Source: three-view drawing plus pictorial views. Frame: mm from the lowest corner of the part. Coordinates: 2 decimals unless noted, no trailing zeros. Loops run counter-clockwise (first coordinate to the right, second up) from the corner with the lowest first, then second, coordinate; pieces in that order, holes last. Notation, with made-up numbers: M -38,-27.5 L -23,-27.5 A20 cw -23,-22.5 Z; hole C 39.5,-6 d11. An arc over 180 degrees is marked long. Use a Markdown table: item, result. Add a question column.
1. Pin query (flat end, axial travel): pin 1 (0.5 mm diameter, centred on x = 79.5, z = 0.5, fed in from -Y). Return the tip coordinate at first contact, or that it passes through.
2. Section B-B on y = 25. Output: boundary loops of the cut face in (x, z).
3. Section C-C on x = 54. Output: boundary loops of the cut face in (y, z), then the cut area to 3 significant figures.
4. Section A-A on z = 0.45. Output: boundary loops of the cut face in (x, y).
5. Line query: L1, parallel to Y at x = 3, z = 0.6; L2, parallel to Y at x = 81, z = 0.15; L3, parallel to Y at x = 14, z = 0.7. Output: solid intervals per line, ascending. Write a range as [from, to].
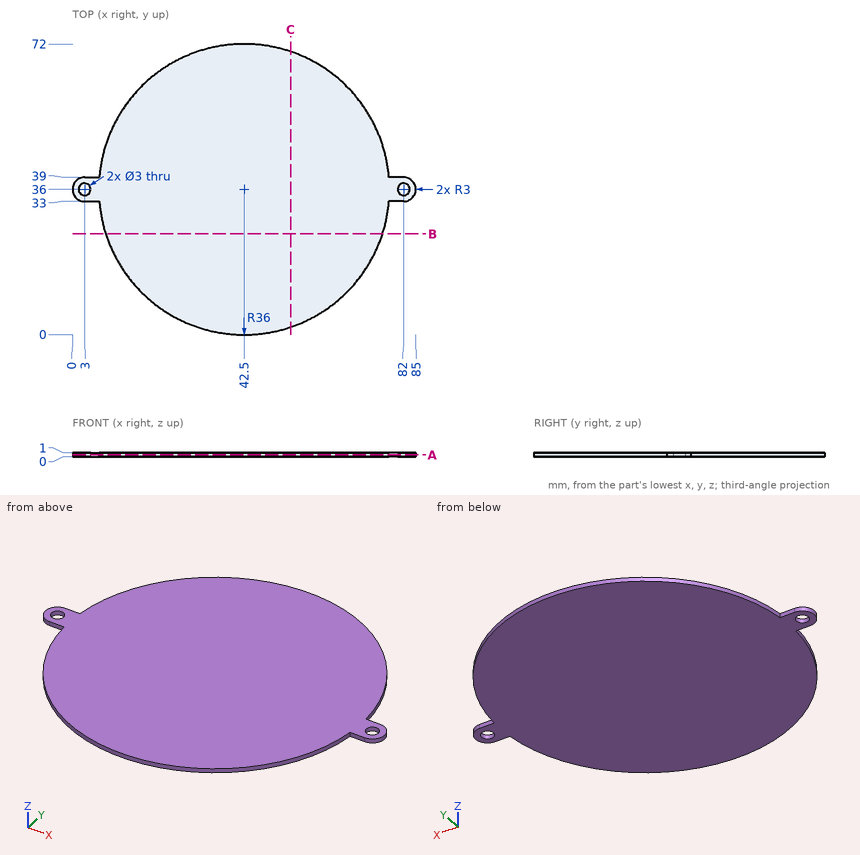
Answers below:
| question | item | result |
|---|---|---|
| 1 | pin 1 | stops at y = 33 |
| 2 | outline | M 8.22,0 L 76.78,0 L 76.78,1 L 8.22,1 Z |
| 3 | outline | M 1.89,0 L 70.11,0 L 70.11,1 L 1.89,1 Z |
| 3 | area | 68.2 mm² |
| 4 | outline | M 3,33 L 6.63,33 A36 ccw 78.37,33 L 82,33 A3 ccw 82,39 L 78.37,39 A36 ccw 6.63,39 L 3,39 A3 ccw Z; hole C 3,36 d3; hole C 82,36 d3 |
| 5 | L1 | y = [33, 34.5], [37.5, 39] |
| 5 | L2 | y = [33, 34.88], [37.12, 39] |
| 5 | L3 | y = [14.01, 57.99] |
